Build history of the part. All positions in model axes, mm. A direction names the side the tool comes from. Coordinates: 2 decimals unless noted, no trailing zeros. Write each loop counter-clockwise with the first axis right and the second up, starting at its lowest first coordinate (ties: lowest second). Pieces come first, ordered by that corner, then holes.
```python
from build123d import *

# Parameters (mm, degrees)
SKETCH1_W           = 70
SKETCH1_H           = 30
SKETCH1_R           = 4.5
SKETCH1_W_2         = 10
SKETCH1_H_2         = 17
BOSS_EXTRUDE1_DEPTH = 2
SKETCH2_W           = 1.5
SKETCH2_H           = 12
BOSS_EXTRUDE2_DEPTH = 8
CUT_EXTRUDE1_REACH  = 40.91
SKETCH3_R           = 1.5
CHAMFER1_SIZE       = 1.7


with BuildPart() as part:
    # Sketch1 → Boss-Extrude1 (new body)
    with BuildSketch(Plane(origin=(0, 0, 0), x_dir=(1, 0, 0), z_dir=(0, 1, 0))):
        Rectangle(SKETCH1_W, SKETCH1_H)
        with Locations(Location((19, 0, 0), (0, 0, 270))):
            Circle(SKETCH1_R, mode=Mode.SUBTRACT)
        with Locations((-17, 0)):
            Rectangle(SKETCH1_W_2, SKETCH1_H_2, mode=Mode.SUBTRACT)
        with Locations((1, 0)):
            Rectangle(SKETCH1_W_2, SKETCH1_H_2, mode=Mode.SUBTRACT)
    extrude(amount=BOSS_EXTRUDE1_DEPTH)

    # Sketch2 → Boss-Extrude2 (add)
    with BuildSketch(Plane(origin=(0, 2, 0), x_dir=(1, 0, 0), z_dir=(0, 1, 0))):
        with Locations((-22.75, 0)):
            Rectangle(SKETCH2_W, SKETCH2_H)
        with Locations((-11.25, 0)):
            Rectangle(SKETCH2_W, SKETCH2_H)
        with Locations((-4.75, 0)):
            Rectangle(SKETCH2_W, SKETCH2_H)
        with Locations((6.75, 0)):
            Rectangle(SKETCH2_W, SKETCH2_H)
        with BuildLine():
            Line((16.938447187, 4), (14.86932209, 4))
            ThreePointArc((14.86932209, 4), (13.25, 0), (14.86932209, -4))
            Line((14.86932209, -4), (16.938447187, -4))
            ThreePointArc((16.938447187, -4), (14.5, 0), (16.938447187, 4))
        make_face()
        with BuildLine():
            Line((23.13067791, 4), (21.061552813, 4))
            ThreePointArc((21.061552813, 4), (22.842329219, 2.342329219), (23.5, 0))
            ThreePointArc((23.5, 0), (22.842329219, -2.342329219), (21.061552813, -4))
            Line((21.061552813, -4), (23.13067791, -4))
            ThreePointArc((23.13067791, -4), (24.75, 0), (23.13067791, 4))
        make_face()
    extrude(amount=BOSS_EXTRUDE2_DEPTH)

    # Sketch3 → Cut-Extrude1 (cut, up to next)
    with BuildSketch(Plane(origin=(0, 2, 0), x_dir=(1, 0, 0), z_dir=(0, 1, 0)), mode=Mode.PRIVATE) as cut_extrude1_sk1:
        with Locations(Location((-31, 11, 0), (0, 0, 270))):
            Circle(SKETCH3_R)
    cut_extrude1_tool1 = extrude(cut_extrude1_sk1.sketch, amount=-CUT_EXTRUDE1_REACH, mode=Mode.PRIVATE) & part.part
    # Sketch3 → Cut-Extrude1 (cut, up to next)
    with BuildSketch(Plane(origin=(0, 2, 0), x_dir=(1, 0, 0), z_dir=(0, 1, 0)), mode=Mode.PRIVATE) as cut_extrude1_sk2:
        with Locations(Location((31, 11, 0), (0, 0, 90))):
            Circle(SKETCH3_R)
    cut_extrude1_tool2 = extrude(cut_extrude1_sk2.sketch, amount=-CUT_EXTRUDE1_REACH, mode=Mode.PRIVATE) & part.part
    # Sketch3 → Cut-Extrude1 (cut, up to next)
    with BuildSketch(Plane(origin=(0, 2, 0), x_dir=(1, 0, 0), z_dir=(0, 1, 0)), mode=Mode.PRIVATE) as cut_extrude1_sk3:
        with Locations(Location((31, -11, 0), (0, 0, 270))):
            Circle(SKETCH3_R)
    cut_extrude1_tool3 = extrude(cut_extrude1_sk3.sketch, amount=-CUT_EXTRUDE1_REACH, mode=Mode.PRIVATE) & part.part
    # Sketch3 → Cut-Extrude1 (cut, up to next)
    with BuildSketch(Plane(origin=(0, 2, 0), x_dir=(1, 0, 0), z_dir=(0, 1, 0)), mode=Mode.PRIVATE) as cut_extrude1_sk4:
        with Locations(Location((-31, -11, 0), (0, 0, 90))):
            Circle(SKETCH3_R)
    cut_extrude1_tool4 = extrude(cut_extrude1_sk4.sketch, amount=-CUT_EXTRUDE1_REACH, mode=Mode.PRIVATE) & part.part
    add(cut_extrude1_tool1.solids().sort_by_distance((-31, 2, -11))[0], mode=Mode.SUBTRACT)
    add(cut_extrude1_tool2.solids().sort_by_distance((31, 2, -11))[0], mode=Mode.SUBTRACT)
    add(cut_extrude1_tool3.solids().sort_by_distance((31, 2, 11))[0], mode=Mode.SUBTRACT)
    add(cut_extrude1_tool4.solids().sort_by_distance((-31, 2, 11))[0], mode=Mode.SUBTRACT)

    # Chamfer1
    chamfer1_edges = [part.edges().sort_by_distance(p)[0] for p in [
        (-31, 0, -12.5),
        (31, 0, -9.5),
        (31, 0, 9.5),
        (-31, 0, 12.5),
    ]]
    chamfer(chamfer1_edges, length=CHAMFER1_SIZE)


solid = part.part
```
1. Saw through at C-C on y = 7.25. List the corners of the cut face in (x, z), plus the area to 3 significant figures.
Computed values:
outline: (-23.5, -6) - (-22, -6) - (-22, 6) - (-23.5, 6) - close; (-12, -6) - (-10.5, -6) - (-10.5, 6) - (-12, 6) - close; (-5.5, -6) - (-4, -6) - (-4, 6) - (-5.5, 6) - close; (6, -6) - (7.5, -6) - (7.5, 6) - (6, 6) - close; (14.87, -4) - (16.94, -4) arc R4.5 cw to (16.94, 4) - (14.87, 4) arc R5.75 ccw to start; (21.06, -4) - (23.13, -4) arc R5.75 ccw to (23.13, 4) - (21.06, 4) arc R4.5 cw to start
area: 95.1 mm2
2. Saw through at B-B on z = 11. List the corners of the cut face in (x, y).
Computed values:
outline: (-35, 0) - (-34.2, 0) - (-32.5, 1.7) - (-32.5, 2) - (-35, 2) - close; (-29.5, 1.7) - (-27.8, 0) - (27.8, 0) - (29.5, 1.7) - (29.5, 2) - (-29.5, 2) - close; (32.5, 1.7) - (34.2, 0) - (35, 0) - (35, 2) - (32.5, 2) - close
3. Mould opens along X. For faces 6 (the face through (-11, 6, 6)), 7 (the face through (13.25, 5.94, -0.06)), 8 (the face through (-23.5, 6, 0)) say: +X half, -X half, draft (parallel to the pull), parting line (faces both ways), or undercut.
Computed values:
face 6: draft
face 7: undercut
face 8: -X half
4. Saw through at A-A on x = 1. List the corners of the cut face in (y, z).
Computed values:
outline: (0, -15) - (2, -15) - (2, -8.5) - (0, -8.5) - close; (0, 8.5) - (2, 8.5) - (2, 15) - (0, 15) - close
5. Probe line 1 along X through (y, z) = (1.95, -11); line 2 along Z through (x, y) = (-15.5, 0.5); line 3 along X through (y, z) = (5, 3). List the from-to ranges inside material, lowest first.
Computed values:
line 1: x = -35 to -32.5, -29.5 to 29.5, 32.5 to 35
line 2: z = -15 to -8.5, 8.5 to 15
line 3: x = -23.5 to -22, -12 to -10.5, -5.5 to -4, 6 to 7.5, 14.09 to 15.65, 22.35 to 23.91
6. Flat gauge pins, fed straight in: pin 1 (1.5 mm diameter, centred on x = -24, y = 6, fed in from -Z); pin 2 (1.2 mm diameter, centred on x = 6.5, y = 7.5, fed in from +Z); pin 3 (3 mm diameter, centred on y = 4, z = -2.5, fed in from -X). Where does each tip first touch, or does it go through?
Computed values:
pin 1: stops at z = -6
pin 2: stops at z = 6
pin 3: stops at x = -23.5
7. Saw through at D-D on x = -31. List the corners of the cut face in (y, z).
Computed values:
outline: (0, -15) - (2, -15) - (2, -12.5) - (1.7, -12.5) - (0, -14.2) - close; (0, -7.8) - (1.7, -9.5) - (2, -9.5) - (2, 9.5) - (1.7, 9.5) - (0, 7.8) - close; (0, 14.2) - (1.7, 12.5) - (2, 12.5) - (2, 15) - (0, 15) - close
8. 3-axis set-ups, long thin cutter, end or side, ignore diameter. For faces 1 (the face through (-11, 6, -6)), 2 (the face through (1, 1, -8.5)), 3 (the face through (-5, 6, 6)), 4 (the face through (0, 1, 15)), 5 (the face through (16, 6, -4)): which of +Z, -Z, +X, -X, +Y, -Y reach the whole face in a straight line?
Computed values:
face 1: -Z, +X, -X, +Y
face 2: +Y, -Y
face 3: +Z, +X, -X, +Y
face 4: +Z, +X, -X, +Y, -Y
face 5: -Z, +X, +Y
